Model file for the job. Use its own axes, mm. A direction names the side the tool comes from. Give positions to 0.01 mm unless a question says otherwise; leave off trailing zeros. Loops run counter-clockwise (first coordinate to the right, second up) from the corner with the lowest first, then second, coordinate; pieces in that order, holes last. Notation, with made-up numbers: (62, 66.5) - (118, 66.5) arc R7 cw to (118, 78.5) - close; hole circle Ø8 at (-29, 49). An arc over 180 degrees is marked (long way). Answer as CSV lines item,"result". Start each with the question number.
Item 1: Saw through at C-C on z = 48. Give the cut face in (x, y), plus the area to 3 significant figures.
Item 2: Saw through at D-D on x = -15.5. Give the cut face in (y, z), plus the area to 3 significant figures.
Item 3: Saw through at A-A on y = 61. Give the cut face in (x, z), plus the area to 3 significant figures.
Item 4: Tool access for faces 4 (the flat face through (-9.151, 48.292, 12.724)), 5 (the flat face through (-20.83, 47.41, 67.2)), 6 (the flat face through (-1.99, 48.29, 15.33)): list every direction of +Z, -Z, +X, -X, +Y, -Y with a clear straight run to the whole face (end or side of a thin tool).
Item 5: Pin check, flat tips, straight feed: pin 1 (6 mm diameter, centred on y = 63.5, z = 53.5, fed in from -X); pin 2 (12 mm diameter, centred on y = 78.5, z = 43, fed in from -X); pin 3 (0.8 mm diameter, centred on y = 47.5, z = 0.5, fed in from +X). Stop position of each tip, or through.
Item 6: Drill centre lines: L1, parallel to Y at x = -8.5, z = 25; L2, parallel to Z at x = -44, y = 81; L3, parallel to Z at x = -8, y = 70.5. Where is each one in solid material? Low to high. Write a range as from..to.
Item 7: Pull direction X, two halves, no side cores. Call faces 1 (the flat face through (-26, 47, 0)), 2 (the flat face through (-16, 2.54, 42)), 3 (the flat face through (-50.8, 47, 1)): pulls with the +X half, pulls with the -X half, needs draft (parallel to the pull), parting line crosses it, or undercut.
Item 8: Saw through at B-B on x = -8.5. Give the cut face in (y, z).
from build123d import *

# Parameters (mm, degrees)
SKETCH1_W           = 95.25
SKETCH1_H           = 50.8
BOSS_EXTRUDE1_DEPTH = 2.54
BOSS_EXTRUDE2_DEPTH = 95.25
SKETCH3_W           = 12.7
SKETCH3_H           = 95.25
BOSS_EXTRUDE3_DEPTH = 2.54
SKETCH4_W           = 12.7
SKETCH4_H           = 95.25
SKETCH4_W_2         = 7.62
SKETCH4_H_2         = 90.17
BOSS_EXTRUDE4_DEPTH = 55.88
CUT_EXTRUDE1_REACH  = 132.474
SKETCH5_W           = 85.09
SKETCH5_H           = 48.26


with BuildPart() as part:
    # Sketch1 → Boss-Extrude1 (new body)
    with BuildSketch(Plane(origin=(0, 0, 0), x_dir=(0, 1, 0), z_dir=(0, 0, 1))):
        with Locations((47.625, 25.4)):
            Rectangle(SKETCH1_W, SKETCH1_H)
    extrude(amount=BOSS_EXTRUDE1_DEPTH)

    # Sketch2 → Boss-Extrude2 (add)
    with BuildSketch(Plane(origin=(0, 95.25, 0), x_dir=(-1, 0, 0), z_dir=(0, 1, 0))):
        Polygon((0, 2.54), (4.34365582, 14.474096284), (6.730475077, 13.60536512), (2.703011542, 2.54), align=None)
    extrude(amount=-BOSS_EXTRUDE2_DEPTH)

    # Sketch3 → Boss-Extrude3 (add)
    with BuildSketch(Plane(origin=(-5.159996085, 0, 14.176972727), x_dir=(0.9396926207859077, 0, 0.34202014332567104), z_dir=(-0.34202014332567104, 0, 0.9396926207859077))):
        with Locations((-0.401268836, 47.625)):
            Rectangle(SKETCH3_W, SKETCH3_H)
    extrude(amount=BOSS_EXTRUDE3_DEPTH)

    # Sketch4 → Boss-Extrude4 (add)
    with BuildSketch(Plane(origin=(-6.028727249, 0, 16.563791984), x_dir=(0.9396926207859075, 0, 0.3420201433256711), z_dir=(-0.3420201433256711, 0, 0.9396926207859075))):
        with Locations((-0.401268836, 47.625)):
            Rectangle(SKETCH4_W, SKETCH4_H)
        with Locations((-0.401268836, 47.625)):
            Rectangle(SKETCH4_W_2, SKETCH4_H_2, mode=Mode.SUBTRACT)
    extrude(amount=BOSS_EXTRUDE4_DEPTH)

    # Sketch5 → Cut-Extrude1 (cut, up to next)
    with BuildSketch(Plane(origin=(5.589978778, 0, 2.034585885), x_dir=(0, 1, 0), z_dir=(0.9396926207859075, 0, 0.3420201433256711)), mode=Mode.PRIVATE) as cut_extrude1_sk1:
        with Locations((47.625, 44.296819257)):
            Rectangle(SKETCH5_W, SKETCH5_H)
    cut_extrude1_tool1 = extrude(cut_extrude1_sk1.sketch, amount=-CUT_EXTRUDE1_REACH, mode=Mode.PRIVATE) & part.part
    add(cut_extrude1_tool1.solids().sort_by_distance((-9.560426, 47.625, 43.65998))[0], mode=Mode.SUBTRACT)


solid = part.part
Responses:
1,outline,"(-24.66, 0) - (-11.14, 0) - (-11.14, 5.08) - (-13.84, 5.08) - (-13.84, 2.54) - (-21.95, 2.54) - (-21.95, 92.71) - (-13.84, 92.71) - (-13.84, 90.17) - (-11.14, 90.17) - (-11.14, 95.25) - (-24.66, 95.25) - close"
1,area,"326 mm2"
2,outline,"(0, 0) - (95.25, 0) - (95.25, 2.54) - (0, 2.54) - close; (0, 22.85) - (95.25, 22.85) - (95.25, 59.98) - (90.17, 59.98) - (90.17, 52.55) - (92.71, 52.55) - (92.71, 30.27) - (2.54, 30.27) - (2.54, 52.55) - (5.08, 52.55) - (5.08, 59.98) - (0, 59.98) - close"
2,area,"1,140 mm2"
3,outline,"(-50.8, 0) - (0, 0) - (0, 2.54) - (-4.34, 14.47) - (0.43, 16.21) - (-1.31, 20.99) - (-3.69, 20.12) - (-2.83, 17.73) - (-9.99, 15.12) - (-29.1, 67.63) - (-31.48, 66.76) - (-11.5, 11.87) - (-6.73, 13.61) - (-2.7, 2.54) - (-50.8, 2.54) - close; (-21.94, 70.24) - (-20.2, 65.47) - (-17.81, 66.33) - (-19.55, 71.11) - close"
3,area,"354 mm2"
4,face 4,"+Y, -Y"
4,face 5,"none"
4,face 6,"+X, +Y, -Y"
5,pin 1,"x = -27.75"
5,pin 2,"x = -25.02"
5,pin 3,"x = 0"
6,L1,"0..2.54, 92.71..95.25"
6,L2,"0..2.54"
6,L3,"0..2.54, 13.14..15.85"
7,face 1,"needs draft"
7,face 2,"undercut"
7,face 3,"pulls with the -X half"
8,outline,"(0, 0) - (95.25, 0) - (95.25, 2.54) - (0, 2.54) - close; (0, 12.96) - (95.25, 12.96) - (95.25, 40.75) - (90.17, 40.75) - (90.17, 33.32) - (92.71, 33.32) - (92.71, 15.66) - (2.54, 15.66) - (2.54, 33.32) - (5.08, 33.32) - (5.08, 40.75) - (0, 40.75) - close"
